Check sheet for the drawn part. Datum: minimum x, y, z corner. Units: mm. A direction names the side the tool comes from. Give positions to 0.01 mm unless a question says otherwise; leave off trailing zeros. Order: outer loops, then holes, each group sorted by start corner. A loop starts at its lowest first (then second) coordinate and runs counter-clockwise, first axis right, second up. Notation, with made-up numbers: (14.25, 21.5) -> (25.25, 21.5) arc R20 ccw to (25.25, 34.5) -> close; hole circle Ø2 at (69.25, 24). An arc over 180 degrees is marked (long way). Return JSON: item names as keys, results as strings. Group by question number.
(1) Cross-section at B-B on x = 50. Enter the section's corners in (y, z), then the cut area to 3 significant figures.
(2) Cross-section at D-D on x = 10.5. Enter the section's corners in (y, z), then the cut area to 3 significant figures.
(3) Cross-section at C-C on y = 40. Enter the section's corners in (x, z) (1 decimal).
(4) Thickness scan on line 1 along Z through (x, y) = (17, 24); line 2 along Y through (x, z) = (55, 59.5); line 3 along Y through (x, z) = (50, 1). Record the ranges inside material, lowest first.
(5) Depth check by flat-ended pin: pin 1 Ø23 at (x, y) = (50, 40) entering from +Z; pin 2 Ø8 at (x, z) = (77, 78.5) entering from +Y; pin 3 Ø16 at (x, y) = (50, 40) entering from -Z. Enter the tip coordinate at first touch or a pass-through.
(6) Tool access check on the marked faces 1 and 2. Record the directions out of +Z, -Z, +X, -X, +Y, -Y that give a thin tool (end or side, any length) a straight path to the whole face; none if there is none.
(7) Cross-section at A-A on y = 5.5. Enter the section's corners in (x, z).
(8) Release check for a two-part mould opening along Z. For the marked faces 3, 4 and 5 record: pulls with the +Z half, pulls with the -Z half, needs draft (parallel to the pull), parting line crosses it, or undercut.
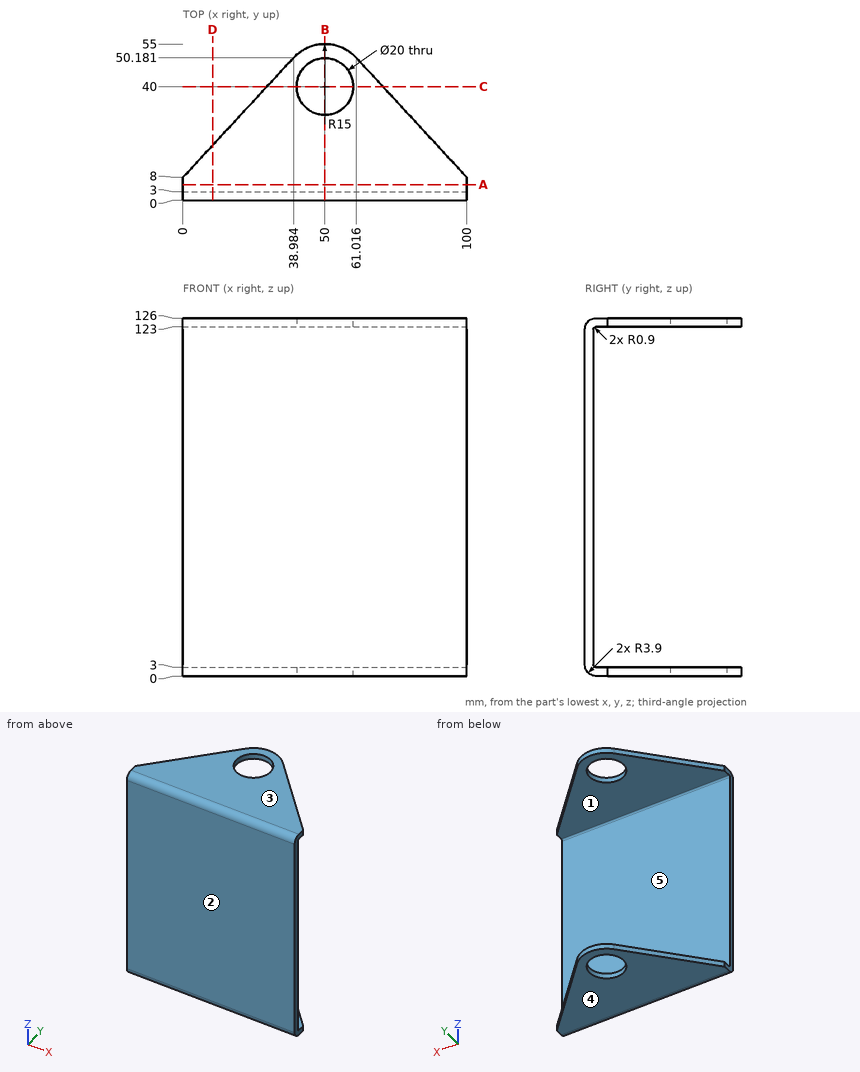
Verdict:
{
 "1": {"outline": "(0, 3.9) arc R3.9 ccw to (3.9, 0) -> (30, 0) -> (30, 3) -> (3.9, 3) arc R0.9 cw to (3, 3.9) -> (3, 122.1) arc R0.9 cw to (3.9, 123) -> (30, 123) -> (30, 126) -> (3.9, 126) arc R3.9 ccw to (0, 122.1) -> close; (50, 0) -> (55, 0) -> (55, 3) -> (50, 3) -> close; (50, 123) -> (55, 123) -> (55, 126) -> (50, 126) -> close", "area": "564 mm²"},
 "2": {"outline": "(0, 3.9) arc R3.9 ccw to (3.9, 0) -> (19.36, 0) -> (19.36, 3) -> (3.9, 3) arc R0.9 cw to (3, 3.9) -> (3, 122.1) arc R0.9 cw to (3.9, 123) -> (19.36, 123) -> (19.36, 126) -> (3.9, 126) arc R3.9 ccw to (0, 122.1) -> close", "area": "470 mm²"},
 "3": {"outline": "(29.6, 0) -> (40, 0) -> (40, 3) -> (29.6, 3) -> close; (29.6, 123) -> (40, 123) -> (40, 126) -> (29.6, 126) -> close; (60, 0) -> (70.4, 0) -> (70.4, 3) -> (60, 3) -> close; (60, 123) -> (70.4, 123) -> (70.4, 126) -> (60, 126) -> close"},
 "4": {"line 1": "0 to 3, 123 to 126", "line 2": "0 to 3", "line 3": "1.29 to 30, 50 to 55"},
 "5": {"pin 1": "z = 126", "pin 2": "y = 3", "pin 3": "through"},
 "6": {"face 1": "+X, -X, +Y", "face 2": "+Z, -Z, +X, -X, -Y"},
 "7": {"outline": "(0, 0) -> (100, 0) -> (100, 3) -> (0, 3) -> close; (0, 123) -> (100, 123) -> (100, 126) -> (0, 126) -> close"},
 "8": {"face 3": "pulls with the +Z half", "face 4": "pulls with the -Z half", "face 5": "undercut"}
}
